Input: part model. Units: mm. Frame: model coordinates. A direction names the side the tool comes from. Coordinates: 2 decimals unless noted, no trailing zeros. Write each loop counter-clockwise with the first axis right and the second up, starting at its lowest first coordinate (ties: lowest second). Pieces come first, ordered by that corner, then holes. Notation, with made-up numbers: (-18, -0.75) - (24, -0.75) arc R20 ccw to (24, 20.25) - close; hole circle Ø1 at (-39.75, -35.75). An arc over 180 degrees is marked (long way). Put each result on its own line as item: value. Start each with the question number.
1. Pin query (flat end, axial travel): pin 1 (1.5 mm diameter, centred on x = -63, z = 112.5, fed in from +Y); pin 2 (8 mm diameter, centred on y = -43.5, z = 61, fed in from +X); pin 3 (5 mm diameter, centred on y = -30.5, z = 89, fed in from -X); pin 4 (21 mm diameter, centred on y = -24.5, z = 13, fed in from -X). Return the tip coordinate at first contact, or that it passes through.
2. Cut plane A-A, the plane y = -32.5. Return loops of the section in (x, z), and give its area (3 significant figures).
3. Access query for faces 1 (the flat face through (-127, -25, -10)), 2 (the flat face through (-110.832, -25, 13)), 3 (the flat face through (-39.095, -25, 128)). Directions: +Z, -Z, +X, -X, +Y, -Y. A direction counts if a zero-diameter tool reaches every point of the face in a straight line with its end or side. Return the directions, or none.
4. Cut plane B-B, the plane x = -23.5. Return loops of the section in (y, z).
5. Line query: line 1 (X direction, y = -37, z = 151); line 2 (Z direction, x = -13, y = -26.5); line 3 (Z direction, x = -90, y = -46.5). Output: solid intervals per line, ascending.
6. Cut plane C-C, the plane z = 102.5. Return loops of the section in (x, y), and give its area (3 significant figures).
from build123d import *

# Parameters (mm, degrees)
F1_DEPTH = 25.4
F4_DEPTH = 25.4
F5_DEPTH = 25.4


# Not quite as in the source:
# - the program builds the solid bodies; features that only make, move or delete a surface that nothing else refers to are left out


with BuildPart() as f1:
    # F0 (on Front) → F1 (new body)
    with BuildSketch(Plane.XZ):
        Polygon((0, -20.290305838), (0, 0), (-19.4481890649, 0), (-110.8317822218, 0), (-127, 0), (-127, -20.290305838), align=None)
        Polygon((-110.8317822218, 0), (-19.4481890649, 0), (-19.4481890649, 26.2184105814), (-25.4435241222, 26.2184105814), (-100.8837223053, 26.2184105814), (-110.8317822218, 26.2184105814), align=None)
        Polygon((-100.8837223053, 26.2184105814), (-25.4435241222, 26.2184105814), (-33.0289951575, 97.0223118013), (-39.0950739384, 97.0021236187), (-39.0950739384, 96.837057952), (-88.6934632531, 96.837057952), (-94.5519953966, 96.8175604939), align=None)
    extrude(amount=F1_DEPTH)

    # F0 (on Front) → F4 (join)
    with BuildSketch(Plane.XZ):
        Polygon((0, -20.290305838), (0, 0), (-19.4481890649, 0), (-110.8317822218, 0), (-127, 0), (-127, -20.290305838), align=None)
        Polygon((-110.8317822218, 0), (-19.4481890649, 0), (-19.4481890649, 26.2184105814), (-25.4435241222, 26.2184105814), (-100.8837223053, 26.2184105814), (-110.8317822218, 26.2184105814), align=None)
        Polygon((-100.8837223053, 26.2184105814), (-25.4435241222, 26.2184105814), (-33.0289951575, 97.0223118013), (-39.0950739384, 97.0021236187), (-39.0950739384, 96.837057952), (-88.6934632531, 96.837057952), (-94.5519953966, 96.8175604939), align=None)
        Polygon((-39.0950739384, 96.837057952), (-39.0950739384, 97.0021236187), (-88.6934632531, 96.837057952), align=None)
        Polygon((-88.6934632531, 96.837057952), (-39.0950739384, 97.0021236187), (-39.0950739384, 160.250261426), (-88.6934632531, 160.250261426), align=None)
    extrude(amount=F4_DEPTH)

    # F0 (on Front) + F4_face (on face) → F5 (join)
    with BuildSketch(Plane.XZ):
        Polygon((0, -20.290305838), (0, 0), (-19.4481890649, 0), (-110.8317822218, 0), (-127, 0), (-127, -20.290305838), align=None)
        Polygon((-110.8317822218, 0), (-19.4481890649, 0), (-19.4481890649, 26.2184105814), (-25.4435241222, 26.2184105814), (-100.8837223053, 26.2184105814), (-110.8317822218, 26.2184105814), align=None)
        Polygon((-100.8837223053, 26.2184105814), (-25.4435241222, 26.2184105814), (-33.0289951575, 97.0223118013), (-39.0950739384, 97.0021236187), (-39.0950739384, 96.837057952), (-88.6934632531, 96.837057952), (-94.5519953966, 96.8175604939), align=None)
        Polygon((-39.0950739384, 96.837057952), (-39.0950739384, 97.0021236187), (-88.6934632531, 96.837057952), align=None)
        Polygon((-88.6934632531, 96.837057952), (-39.0950739384, 97.0021236187), (-39.0950739384, 160.250261426), (-88.6934632531, 160.250261426), align=None)
    with BuildSketch(Plane(origin=(-63.8821440169, -25.4, 54.1439890392), x_dir=(1, 0, 0), z_dir=(0, -1, 0))):
        Polygon((63.8821440169, -74.4342948772), (63.8821440169, -54.1439890392), (44.433954952, -54.1439890392), (44.433954952, -27.9255784579), (38.4386198947, -27.9255784579), (30.8531488594, 42.8783227621), (24.7870700785, 42.8581345795), (24.7870700785, 106.1062723867), (-24.8113192362, 106.1062723867), (-24.8113192362, 42.6930689128), (-30.6698513797, 42.6735714547), (-37.0015782884, -27.9255784579), (-46.9496382049, -27.9255784579), (-46.9496382049, -54.1439890392), (-63.1178559831, -54.1439890392), (-63.1178559831, -74.4342948772), align=None)
    extrude(amount=F5_DEPTH)


solid = f1.part
Report:
1. pin 1: stops at y = 0
1. pin 2: stops at x = -28.74
1. pin 3: stops at x = -95.48
1. pin 4: stops at x = -110.83
2. outline: (-127, -20.29) - (0, -20.29) - (0, 0) - (-19.45, 0) - (-19.45, 26.22) - (-25.44, 26.22) - (-33.03, 97.02) - (-39.1, 97) - (-39.1, 160.25) - (-88.69, 160.25) - (-88.69, 96.84) - (-94.55, 96.82) - (-100.88, 26.22) - (-110.83, 26.22) - (-110.83, 0) - (-127, 0) - close
2. area: 13,000 mm^2
3. face 1: +Z, -Z, -X, +Y, -Y
3. face 2: +Z, -X, +Y, -Y
3. face 3: +Z, +X, +Y, -Y
4. outline: (-50.8, -20.29) - (0, -20.29) - (0, 26.22) - (-50.8, 26.22) - close
5. line 1: x = -88.69 to -39.1
5. line 2: z = -20.29 to 0
5. line 3: z = -20.29 to 96.83
6. outline: (-88.69, -50.8) - (-39.1, -50.8) - (-39.1, 0) - (-88.69, 0) - close
6. area: 2,520 mm^2
